Autodesk Inventor part; units mm, degrees
ref_plane "YZ Plane" through (0, 0, 0) normal (1, 0, 0) x (0, 1, 0)
ref_plane "XZ Plane" through (0, 0, 0) normal (0, 1, 0) x (-1, 0, 0)
ref_plane "XY Plane" through (0, 0, 0) normal (0, 0, 1) x (1, 0, 0)
sketch "스케치1" plane through (0, 0, 0) normal (0, 0, 1) x (1, 0, 0)
  line L0 (0, 0) -> (18.6, 0)
  line L1 (18.6, 0) -> (18.6, 13.5)
  line L2 (18.6, 13.5) -> (0, 13.5)
  line L3 (0, 13.5) -> (0, 0)
  line L4 (1.5, 12) -> (17.1, 12)
  line L5 (17.1, 12) -> (17.1, 1.5)
  line L6 (17.1, 1.5) -> (1.5, 1.5)
  line L7 (1.5, 1.5) -> (1.5, 12)
  dimension "d4" = 18.6
  dimension "d5" = 13.5
  dimension "d6" = 1.5
extrude "돌출1" add sketch "스케치1" along normal blind 25.5
sketch "스케치2" plane through (0, 0, 25.5) normal (0, 0, 1) x (1, 0, 0)
  line L0 (0, 0) -> (18.6, 0)
  line L1 (18.6, 0) -> (18.6, 13.5)
  line L2 (0, 0) -> (18.6, 0)
  line L3 (18.6, 0) -> (18.6, 8)
  line L4 (18.6, 8) -> (0, 8)
  line L5 (18.6, 13.5) -> (0, 13.5)
  line L6 (18.6, 8) -> (10.6, 8)
  line L7 (10.6, 8) -> (10.6, 13.5)
  line L8 (10.6, 13.5) -> (18.6, 13.5)
  line L9 (18.6, 13.5) -> (18.6, 8)
  line L10 (0, 13.5) -> (0, 0)
  line L11 (17.1, 12) -> (1.5, 12)
  line L12 (0, 13.5) -> (10.6, 13.5)
  line L13 (10.6, 13.5) -> (10.6, 12)
  line L14 (10.6, 12) -> (0, 12)
  line L15 (0, 12) -> (0, 13.5)
  line L16 (1.5, 1.5) -> (1.5, 12)
  line L17 (7.5, 8) -> (7.5, 0)
  point P0 (0, 12)
  dimension "d9" = 8
  dimension "d14" = 8
  dimension "d58" = 6
extrude "돌출2" add sketch "스케치2" along normal blind 1 contours L17 L4 L1 L0 | L10 L5 L7 L11 L14 | L4 L7 L5 L1
sketch "스케치3" plane through (0, 0, 0) normal (0, 0, -1) x (-1, 0, 0)
  line L0 (-17.1, 1.5) -> (-17.1, 12)
  line L1 (-17.1, 12) -> (-1.5, 12)
  line L2 (-1.5, 12) -> (-1.5, 1.5)
  line L3 (-1.5, 1.5) -> (-17.1, 1.5)
  line L4 (0, 0) -> (-18.6, 0)
  line L5 (0, 13.5) -> (0, 0)
  line L6 (-18.6, 13.5) -> (0, 13.5)
  line L7 (-18.6, 0) -> (-18.6, 13.5)
  line L8 (-18.6, 13.5) -> (0, 13.5)
  line L9 (0, 0) -> (-1.5, 0)
  line L10 (-1.5, 0) -> (-1.5, 13.5)
  line L11 (-1.5, 13.5) -> (0, 13.5)
  line L12 (0, 13.5) -> (0, 0)
  point P0 (-1.5, 6.75)
extrude "돌출3" cut sketch "스케치3" against normal up to next contours L2 L10 L6 L5 L4
sketch "스케치4" plane through (18.6, 0, 0) normal (0, -1, 0) x (1, 0, 0)
  line L0 (-7.8, 21) -> (-17.1, 21)
  line L1 (-17.1, 21) -> (-17.1, 21.5)
  line L2 (-17.1, 21.5) -> (-7.8, 21.5)
  line L3 (-7.8, 21.5) -> (-7.8, 21)
  line L4 (-17.1, 25.5) -> (-17.1, 0)
  line L5 (-11.1, 26.5) -> (0, 26.5)
  point P0 (-18.6, 0)
  point P1 (-17.1, 26.5)
  dimension "d17" = 0.5
  dimension "d18" = 9.3
  dimension "d19" = 5
extrude "돌출4" cut sketch "스케치4" against normal up to next
fillet "모깎기1" radius 1 2 edges at (18.6, 13.5, 13.25) (18.6, 0, 13.25)
sketch "스케치11" plane through (1.5, 12, 0) normal (-1, 0, 0) x (0, 0, 1)
  line L0 (1, 0.75) -> (2, 0.75)
  line L1 (2, 0.75) -> (2, -11.25)
  line L2 (2, -11.25) -> (1, -11.25)
  line L3 (1, -11.25) -> (1, 0.75)
  line L4 (0, -10.5) -> (0, 0)
  line L5 (0, 1.5) -> (26.5, 1.5)
  line L6 (21, -12) -> (0, -12)
  dimension "d43" = 1
  dimension "d44" = 1
  dimension "d45" = 0.75
  dimension "d46" = 0.75
extrude "돌출8" cut sketch "스케치11" against normal blind 16.1
equation "\"d6\" = t"
equation "\"t\" = 1.5"
properties part number "_3D 인쇄"
Build history of the part. All positions in model axes, mm. A direction names the side the tool comes from. Round coordinates to 2 decimals unless told otherwise and drop trailing zeros. Order: outer loops, then holes, each group sorted by start corner. A loop starts at its lowest first (then second) coordinate and runs counter-clockwise, first axis right, second up. Notation, with made-up numbers: (63.25, 47.5) - (80.25, 47.5) arc R17 ccw to (80.25, 57.5) - close; hole circle Ø1 at (61.5, 10.5). An arc over 180 degrees is marked (long way). Use a Markdown table: item, result.
1) Saw through at C-C on z = 17.5. Write the cut outline in (x, y), and give its area (3 significant figures).
Recorded:
| item | result |
|---|---|
| outline | (1.5, 0) - (17.6, 0) arc R1 ccw to (18.6, 1) - (18.6, 12.5) arc R1 ccw to (17.6, 13.5) - (1.5, 13.5) - (1.5, 12) - (17.1, 12) - (17.1, 1.5) - (1.5, 1.5) - close |
| area | 66.6 mm² |
2) Saw through at B-B on y = 9.25. Write the cut outline in (x, z).
Recorded:
| item | result |
|---|---|
| outline | (10.6, 25.5) - (17.1, 25.5) - (17.1, 2) - (17.6, 2) - (17.6, 1) - (17.1, 1) - (17.1, 0) - (18.6, 0) - (18.6, 26.5) - (10.6, 26.5) - close |
3) Wall check: L1, parallel to Y at x = 7, z = 17.25; L2, parallel to Y at x = 10.25, z = 1.5; L3, parallel to Z at x = 17.25, y = 1.25. Give the ranges that are in metal, low to high.
Recorded:
| item | result |
|---|---|
| L1 | y = 0 to 1.5, 12 to 13.5 |
| L2 | y = 0 to 0.75, 12.75 to 13.5 |
| L3 | z = 0 to 1, 2 to 26.5 |
4) Saw through at D-D on x = 8.25. Write the cut outline in (y, z).
Recorded:
| item | result |
|---|---|
| outline | (0, 0) - (1.5, 0) - (1.5, 1) - (0.75, 1) - (0.75, 2) - (1.5, 2) - (1.5, 21) - (0, 21) - close; (0, 21.5) - (1.5, 21.5) - (1.5, 25.5) - (8, 25.5) - (8, 26.5) - (0, 26.5) - close; (12, 0) - (13.5, 0) - (13.5, 26.5) - (12, 26.5) - (12, 2) - (12.75, 2) - (12.75, 1) - (12, 1) - close |
5) Saw through at A-A on x = 5. Write the cut outline in (y, z), and give its area (4 significant figures).
Recorded:
| item | result |
|---|---|
| outline | (0, 0) - (1.5, 0) - (1.5, 1) - (0.75, 1) - (0.75, 2) - (1.5, 2) - (1.5, 21) - (0, 21) - close; (0, 21.5) - (1.5, 21.5) - (1.5, 25.5) - (0, 25.5) - close; (12, 0) - (13.5, 0) - (13.5, 26.5) - (12, 26.5) - (12, 2) - (12.75, 2) - (12.75, 1) - (12, 1) - close |
| area | 75.75 mm² |
6) Pull direction Y, two halves, no side cores. Call faces 4 (the face through (9.4, 1.5, 0.5)), 5 (the face through (18.299, 0.285, 13.436)), 6 (the face through (12, 7, 26.5)): pulls with the +Y half, pulls with the -Y half, needs draft (parallel to the pull), parting line crosses it, or undercut.
Recorded:
| item | result |
|---|---|
| face 4 | undercut |
| face 5 | pulls with the -Y half |
| face 6 | needs draft |
7) Flat gauge pins, fed straight in: pin 1 Ø1.2 at (x, y) = (5.5, 1) entering from -Z; pin 2 Ø3 at (y, z) = (4.5, 10) entering from -X; pin 3 Ø1.6 at (x, y) = (6, 1) entering from +Z; pin 4 Ø2 at (x, y) = (11, 4.5) entering from -Z. Where does each tip first touch, or does it go through?
Recorded:
| item | result |
|---|---|
| pin 1 | stops at z = 0 |
| pin 2 | stops at x = 17.1 |
| pin 3 | stops at z = 25.5 |
| pin 4 | stops at z = 25.5 |
8) Tool access for faces 1 (the face through (11, 1, 1)), 2 (the face through (6, 1, 21.5)), 3 (the face through (4, 1, 25.5)): list every direction of +Z, -Z, +X, -X, +Y, -Y with a clear straight run to the whole face (end or side of a thin tool).
Recorded:
| item | result |
|---|---|
| face 1 | -X |
| face 2 | -X, -Y |
| face 3 | +Z, -X, -Y |
